Source: CAD feature listing. Evaluate the final solid. Frame: model axes, mm. Face numbers are marked on the shaded views. A direction names the side the tool comes from. Coordinates: 2 decimals unless noted, no trailing zeros. Write each loop counter-clockwise with the first axis right and the second up, starting at its lowest first coordinate (ties: lowest second). Pieces come first, ordered by that corner, then holes. Notation, with made-up numbers: (-24, 50) -> (29, 50) arc R13 cw to (29, 67) -> close; hole circle Ø7 at (31, -29). An arc over 180 degrees is marked (long way). One line per item, written item: value. Start each with the question number.
1. Line query: line 1 (X direction, y = 67, z = 0.55); line 2 (X direction, y = 4, z = -6); line 3 (Z direction, x = -13, y = 8.5). Output: solid intervals per line, ascending.
2. Mould query, pull axis Z, two halves, no side actions, for the marked faces 1, 2, 3 and 4. Classes: released by +Z, released by -Z, zero draft, split by the parting line, or undercut.
3. Section query A-A, the plane z = -10. Output: boundary loops of the cut face in (x, y), and give its area (3 significant figures).
4. First-contact query: P1, Ø5, axis at x = 9, z = -6, coming from the -Y side; P2, Ø1, axis at x = -14.5, y = 58.5, coming from the -Z side; P3, Ø3, axis at x = 19, z = -9, coming from the -Y side. Flat tips, straight axial feed; report the tip coordinate or a pass-through.
5. Access query for the marked faces 5 and 6. Directions: +Z, -Z, +X, -X, +Y, -Y. A direction counts if a zero-diameter tool reaches every point of the face in a straight line with its end or side. Return the directions, or none.
6. Section query B-B, the plane y = -9. Output: boundary loops of the cut face in (x, z), and give its area (3 significant figures).
7. Section query C-C, the plane y = 45. Output: boundary loops of the cut face in (x, z).
from build123d import *

# Parameters (mm, degrees)
SKETCH1_R                      = 1.35
BASE_FLANGE1_DEPTH             = 0.8
EDGE_FLANGE1_STRIP_W           = 7.2
EDGE_FLANGE1_STRIP_H           = 0.8
EDGE_FLANGE1_STRIP_CUT_DEPTH   = 50
EDGE_FLANGE1_STRIP_2_W         = 7.2
EDGE_FLANGE1_STRIP_2_H         = 0.8
EDGE_FLANGE1_STRIP_CUT_2_DEPTH = 55.5
EDGE_FLANGE1_DEPTH             = 50
EDGE_FLANGE1_BEND_DEPTH        = 55.5
EDGE_FLANGE4_DEPTH             = 10.5
EDGE_FLANGE4_BEND_DEPTH        = 10.5
EDGE_FLANGE5_DEPTH             = 50
EDGE_FLANGE5_BEND_DEPTH        = 55.5


# Sheet-metal steps are written as plain solids
with BuildPart() as part:
    # Sketch1 → Base-Flange1 (new body)
    with BuildSketch(Plane.XY):
        Polygon((15.25, 0), (15.25, -12), (-15.25, -12), (-15.25, -5.5), (-21.25, -5.5), (-21.25, 50), (-15.25, 50), (-15.25, 70), (15.25, 70), (15.25, 50), (21.25, 50), (21.25, 0), align=None)
        with Locations((8.737756115, -9)):
            Circle(SKETCH1_R, mode=Mode.SUBTRACT)
        with Locations((-5.262243885, -9)):
            Circle(SKETCH1_R, mode=Mode.SUBTRACT)
        with Locations((8.737756115, 67)):
            Circle(SKETCH1_R, mode=Mode.SUBTRACT)
        with Locations((-5.262243885, 67)):
            Circle(SKETCH1_R, mode=Mode.SUBTRACT)
    extrude(amount=BASE_FLANGE1_DEPTH)

    # Edge-Flange1 strip (across the edge) → Edge-Flange1 strip cut (cut)
    with BuildSketch(Plane(origin=(21.25, 50, 0), x_dir=(-1, 0, 0), z_dir=(0, -1, 0))):
        with Locations((-1.6, -0.4)):
            Rectangle(EDGE_FLANGE1_STRIP_W, EDGE_FLANGE1_STRIP_H)
    extrude(amount=EDGE_FLANGE1_STRIP_CUT_DEPTH, mode=Mode.SUBTRACT)

    # Edge-Flange1 strip 2 (across the edge) → Edge-Flange1 strip cut 2 (cut)
    with BuildSketch(Plane(origin=(-21.25, -5.5, 0), x_dir=(1, 0, 0), z_dir=(0, 1, 0))):
        with Locations((-1.6, -0.4)):
            Rectangle(EDGE_FLANGE1_STRIP_2_W, EDGE_FLANGE1_STRIP_2_H)
    extrude(amount=EDGE_FLANGE1_STRIP_CUT_2_DEPTH, mode=Mode.SUBTRACT)

    # Edge-Flange1 section (across the edge) → Edge-Flange1 (add)
    with BuildSketch(Plane(origin=(21.25, 50, 0), x_dir=(-1, 0, 0), z_dir=(0, -1, 0))):
        with BuildLine():
            Line((-0.8, 2), (-0.8, 12.5))
            Line((-0.8, 12.5), (0, 12.5))
            Line((0, 12.5), (0, 2))
            ThreePointArc((0, 2), (0.585786438, 0.585786438), (2, 0))
            Line((2, 0), (2, -0.8))
            ThreePointArc((2, -0.8), (0.020101013, 0.020101013), (-0.8, 2))
        make_face()
    extrude(amount=EDGE_FLANGE1_DEPTH)

    # Edge-Flange1 section 2 (across the edge) → Edge-Flange1 bend (add)
    with BuildSketch(Plane(origin=(-21.25, -5.5, 0), x_dir=(1, 0, 0), z_dir=(0, 1, 0))):
        with BuildLine():
            Line((-0.8, 2), (-0.8, 12.5))
            Line((-0.8, 12.5), (0, 12.5))
            Line((0, 12.5), (0, 2))
            ThreePointArc((0, 2), (0.585786438, 0.585786438), (2, 0))
            Line((2, 0), (2, -0.8))
            ThreePointArc((2, -0.8), (0.020101013, 0.020101013), (-0.8, 2))
        make_face()
    extrude(amount=EDGE_FLANGE1_BEND_DEPTH)

    # Edge-Flange4 section (across the edge) → Edge-Flange4 (add)
    with BuildSketch(Plane(origin=(21.25, 52, -2), x_dir=(0, -1, 0), z_dir=(0, 0, -1))):
        with BuildLine():
            Line((-0.8, 2), (-0.8, 20))
            Line((-0.8, 20), (0, 20))
            Line((0, 20), (0, 2))
            ThreePointArc((0, 2), (0.585786438, 0.585786438), (2, 0))
            Line((2, 0), (2, -0.8))
            ThreePointArc((2, -0.8), (0.020101013, 0.020101013), (-0.8, 2))
        make_face()
    extrude(amount=EDGE_FLANGE4_DEPTH)

    # Edge-Flange4 section 2 (across the edge) → Edge-Flange4 bend (add)
    with BuildSketch(Plane(origin=(-21.25, 52, -12.5), x_dir=(0, -1, 0), z_dir=(0, 0, 1))):
        with BuildLine():
            Line((-0.8, 2), (-0.8, 20))
            Line((-0.8, 20), (0, 20))
            Line((0, 20), (0, 2))
            ThreePointArc((0, 2), (0.585786438, 0.585786438), (2, 0))
            Line((2, 0), (2, -0.8))
            ThreePointArc((2, -0.8), (0.020101013, 0.020101013), (-0.8, 2))
        make_face()
    extrude(amount=EDGE_FLANGE4_BEND_DEPTH)

    # Edge-Flange5 section (across the edge) → Edge-Flange5 (add)
    with BuildSketch(Plane(origin=(21.25, 50, -14.5), x_dir=(0, 0, 1), z_dir=(0, -1, 0))):
        with BuildLine():
            Line((-0.8, 2), (-0.8, 10))
            Line((-0.8, 10), (0, 10))
            Line((0, 10), (0, 2))
            ThreePointArc((0, 2), (0.585786438, 0.585786438), (2, 0))
            Line((2, 0), (2, -0.8))
            ThreePointArc((2, -0.8), (0.020101013, 0.020101013), (-0.8, 2))
        make_face()
    extrude(amount=EDGE_FLANGE5_DEPTH)

    # Edge-Flange5 section 2 (across the edge) → Edge-Flange5 bend (add)
    with BuildSketch(Plane(origin=(-21.25, -5.5, -14.5), x_dir=(0, 0, 1), z_dir=(0, 1, 0))):
        with BuildLine():
            Line((-0.8, 2), (-0.8, 10))
            Line((-0.8, 10), (0, 10))
            Line((0, 10), (0, 2))
            ThreePointArc((0, 2), (0.585786438, 0.585786438), (2, 0))
            Line((2, 0), (2, -0.8))
            ThreePointArc((2, -0.8), (0.020101013, 0.020101013), (-0.8, 2))
        make_face()
    extrude(amount=EDGE_FLANGE5_BEND_DEPTH)


solid = part.part
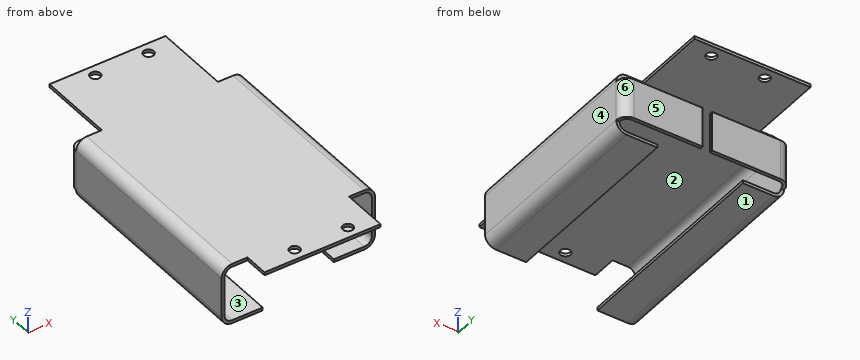
Computed values:
1. line 1: x = -15.25 to -6.61, -3.91 to 7.39, 10.09 to 15.25
1. line 2: x = -22.05 to -21.25, 21.25 to 22.05
1. line 3: z = -15.3 to -14.5, 0 to 0.8
2. face 1: released by -Z
2. face 2: undercut
2. face 3: undercut
2. face 4: zero draft
3. outline: (-22.05, -5.5) -> (-21.25, -5.5) -> (-21.25, 50) arc R2 cw to (-19.25, 52) -> (-1.25, 52) -> (-1.25, 52.8) -> (-19.25, 52.8) arc R2.8 ccw to (-22.05, 50) -> close; (1.25, 52) -> (19.25, 52) arc R2 cw to (21.25, 50) -> (21.25, 0) -> (22.05, 0) -> (22.05, 50) arc R2.8 ccw to (19.25, 52.8) -> (1.25, 52.8) -> close
3. area: 119 mm²
4. P1: stops at y = 52
4. P2: stops at z = 0
4. P3: stops at y = 51.56
5. face 5: -Z, +X, -X, +Y
5. face 6: +Z, -Z, +X, +Y
6. outline: (-15.25, 0) -> (-6.61, 0) -> (-6.61, 0.8) -> (-15.25, 0.8) -> close; (-3.91, 0) -> (7.39, 0) -> (7.39, 0.8) -> (-3.91, 0.8) -> close; (10.09, 0) -> (15.25, 0) -> (15.25, 0.8) -> (10.09, 0.8) -> close
6. area: 20.1 mm²
7. outline: (-22.05, -12.5) arc R2.8 ccw to (-19.25, -15.3) -> (-11.25, -15.3) -> (-11.25, -14.5) -> (-19.25, -14.5) arc R2 cw to (-21.25, -12.5) -> (-21.25, -2) arc R2 cw to (-19.25, 0) -> (19.25, 0) arc R2 cw to (21.25, -2) -> (21.25, -12.5) arc R2 cw to (19.25, -14.5) -> (11.25, -14.5) -> (11.25, -15.3) -> (19.25, -15.3) arc R2.8 ccw to (22.05, -12.5) -> (22.05, -2) arc R2.8 ccw to (19.25, 0.8) -> (-19.25, 0.8) arc R2.8 ccw to (-22.05, -2) -> close
